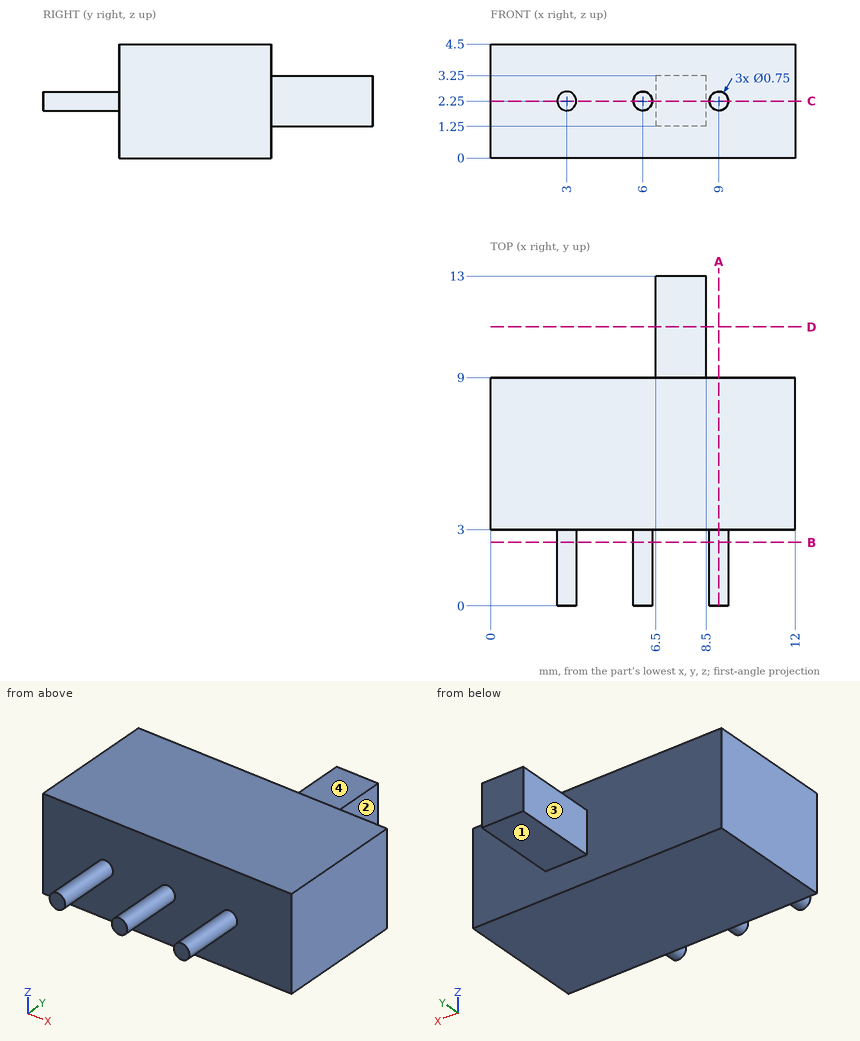
The drawing under review shows one solid part. Ordinate dimensions are in mm from its lowest x, y, z. A direction names the side the tool comes from. Give positions to 0.01 mm unless a question says otherwise; leave off trailing zeros. Loops run counter-clockwise (first coordinate to the right, second up) from the corner with the lowest first, then second, coordinate; pieces in that order, holes last. Notation, with made-up numbers: M 79,-30.5 L 132,-30.5 A15 ccw 132,-3.5 Z; hole C -31,39 d8. An arc over 180 degrees is marked long. Return JSON: item names as keys, results as strings. Group by question number.
Item 1: We need section D-D (y = 11). Give the boundary of the cut face in (x, z), and give its area (3 significant figures).
Item 2: Insertion check: pin 1 Ø3 at (x, y) = (4, 8) entering from -Z; pin 2 Ø0.6 at (y, z) = (11, 2) entering from +X; pin 3 Ø1 at (x, y) = (7.5, 11) entering from +Z; pin 4 Ø0.6 at (x, y) = (7, 12) entering from -Z. Each pin has a flat end and moves straight along its axis. Give the tip position at first contact, or say it passes through.
Item 3: We need section B-B (y = 2.5). Give the boundary of the cut face in (x, z) (3 decimals).
Item 4: Tool access review of the marked faces 1, 2, 3 and 4: name each direction out of +Z, -Z, +X, -X, +Y, -Y from which nothing blocks a thin tool from reaching the whole face with its end or side.
Item 5: We need section C-C (z = 2.25). Give the boundary of the cut face in (x, y) (3 decimals), and give its area (4 significant figures).
Item 6: For probe 1 along Y at (x, z) = (9, 4); probe 2 along X at (y, z) = (9.75, 3.2); probe 3 along Y at (x, z) = (7.25, 2.35), list the stretches that pass through material, from the lowest coordinate up.
Item 7: We need section A-A (x = 9). Give the boundary of the cut face in (y, z) (3 decimals), and give its area (4 significant figures).
Output:
{
 "1": {"outline": "M 6.5,1.25 L 8.5,1.25 L 8.5,3.25 L 6.5,3.25 Z", "area": "4.00 mm^2"},
 "2": {"pin 1": "stops at z = 0", "pin 2": "stops at x = 8.5", "pin 3": "stops at z = 3.25", "pin 4": "stops at z = 1.25"},
 "3": {"outline": "C 3,2.25 d0.75; C 6,2.25 d0.75; C 9,2.25 d0.75"},
 "4": {"face 1": "-Z, +X, -X, +Y", "face 2": "+Z, -Z, +X, +Y", "face 3": "+Z, -Z, -X, +Y", "face 4": "+Z, +X, -X, +Y"},
 "5": {"outline": "M 0,3 L 2.625,3 L 2.625,0 L 3.375,0 L 3.375,3 L 5.625,3 L 5.625,0 L 6.375,0 L 6.375,3 L 8.625,3 L 8.625,0 L 9.375,0 L 9.375,3 L 12,3 L 12,9 L 8.5,9 L 8.5,13 L 6.5,13 L 6.5,9 L 0,9 Z", "area": "86.75 mm^2"},
 "6": {"probe 1": "y = 3 to 9", "probe 2": "x = 6.5 to 8.5", "probe 3": "y = 3 to 13"},
 "7": {"outline": "M 0,1.875 L 3,1.875 L 3,0 L 9,0 L 9,4.5 L 3,4.5 L 3,2.625 L 0,2.625 Z", "area": "29.25 mm^2"}
}
